The listing builds one solid part. Answer for the finished solid, in the listing's coordinates (mm). A direction names the side the tool comes from. Give positions to 0.01 mm unless a question says otherwise; leave off trailing zeros. Loops run counter-clockwise (first coordinate to the right, second up) from the corner with the lowest first, then second, coordinate; pieces in that order, holes last. Notation, with made-up numbers: M 7.5,-33.5 L 62.5,-33.5 A33 cw 62.5,-4.5 Z; hole C 88.5,-14 d3. An arc over 180 degrees is marked long. Use one line per item in the form item = value. Start each with the question number.
1. For faces 1 (the face through (6.29, 3.13, 4.41)), 2 (the face through (20, 10, 0)), determine the directions among +Z, -Z, +X, -X, +Y, -Y from which every point of the face is accessible in a straight line to the end or side of a thin tool.
2. The part is cut by section C-C (x = 20). Write down the section's boundary in (y, z) (3 decimals), and give its area (3 significant figures).
3. The part is cut by section A-A (z = 4). Write down the section's boundary in (x, y) (3 decimals).
4. Straight lines are drawn through the part: line 1 (Y direction, x = 20, z = 5.75) (3 decimals); line 2 (Z direction, x = 35, y = 2.25); line 3 (Y direction, x = 21, z = 1.25). For each, find the intervals that lie inside material, in ascending order. Write a range as from..to.
5. The part is cut by section B-B (y = 12.7). Write down the section's boundary in (x, z) (3 decimals), and give its area (3 significant figures).
6. The part is cut by section D-D (x = 35). Write down the section's boundary in (y, z), and give its area (3 significant figures).
7. The mould has two halves that part along X. Classify faces 3 (the face through (20, 10, 8)), 4 (the face through (35, 6.35, 4)), 5 (the face through (40, 13, 4)): released by +X, released by -X, zero draft, split by the parting line, or undercut.
8. This flat-tipped pin is pushed along its axis until it touches: pin 1 Ø1.4 at (x, z) = (4.5, 4) entering from -Y. Where does it stop, or does it pass through?
from build123d import *

# Parameters (mm, degrees)
F0_W     = 40
F0_H     = 25.4
F1_DEPTH = 8
F3_R     = 1.35255
F4_DEPTH = 6.35
F2_R     = 1.625
F5_DEPTH = 25.4


with BuildPart() as f1:
    # F0 (on Top) → F1 (new body)
    with BuildSketch(Plane.XY):
        with Locations((20, 12.7)):
            Rectangle(F0_W, F0_H)
    extrude(amount=F1_DEPTH)

    # F3 (on face) → F4 (cut)
    with BuildSketch(Plane.XZ):
        with Locations((5, 4)):
            Circle(F3_R)
        with Locations((35, 4)):
            Circle(F3_R)
    extrude(amount=-F4_DEPTH, mode=Mode.SUBTRACT)

    # F2 (on face) → F5 (cut)
    with BuildSketch(Plane.XY.offset(8)):
        with Locations((20, 12.7)):
            Circle(F2_R)
    extrude(amount=-F5_DEPTH, mode=Mode.SUBTRACT)


solid = f1.part
Derived:
q1.face_1 = -Y
q1.face_2 = -Z, +X, -X, +Y, -Y
q2.outline = M 0,0 L 11.075,0 L 11.075,8 L 0,8 Z; M 14.325,0 L 25.4,0 L 25.4,8 L 14.325,8 Z
q2.area = 177 mm2
q3.outline = M 0,0 L 3.647,0 L 3.647,6.35 L 6.353,6.35 L 6.353,0 L 33.647,0 L 33.647,6.35 L 36.353,6.35 L 36.353,0 L 40,0 L 40,25.4 L 0,25.4 Z; hole C 20,12.7 d3.25
q4.line_1 = 0..11.075, 14.325..25.4
q4.line_2 = 0..2.65, 5.35..8
q4.line_3 = 0..11.42, 13.98..25.4
q5.outline = M 0,0 L 18.375,0 L 18.375,8 L 0,8 Z; M 21.625,0 L 40,0 L 40,8 L 21.625,8 Z
q5.area = 294 mm2
q6.outline = M 0,0 L 25.4,0 L 25.4,8 L 0,8 L 0,5.35 L 6.35,5.35 L 6.35,2.65 L 0,2.65 Z
q6.area = 186 mm2
q7.face_3 = zero draft
q7.face_4 = undercut
q7.face_5 = released by +X
q8.pin_1 = 6.35
